For this review, take the finished solid that the model builds, in its own axes (mm). Coordinates: 2 decimals unless noted, no trailing zeros. Loops run counter-clockwise (first coordinate to the right, second up) from the corner with the lowest first, then second, coordinate; pieces in that order, holes last.
1. Take a section at A-A, the plane x = 3.4. State the section outline as (y, z) points, then the cut area to 3 significant figures.
2. Take a section at C-C, the plane y = 2.5. State the section outline as (x, z) points.
3. Clearance check with flat-ended pins moving along their axes: P1, Ø1, axis at y = -34.5, z = 51.5, coming from the -X side; P2, Ø1.5, axis at y = -28, z = -3.5, coming from the -X side; P3, Ø1.4, axis at x = 2, z = -3.5, coming from the +Y side; P4, Ø1.4, axis at x = 3, z = -2, coming from the -Y side. State where each tip first meets the part, or that it passes through.
4. Take a section at D-D, the plane y = 20.5. State the section outline as (x, z) points.
5. Take a section at B-B, the plane z = 77. State the section outline as (x, y) points, then the cut area to 3 significant figures.
6. To check wall thickness, follow probe 1 along Z at (x, y) = (2.8, 0); probe 2 along Z at (x, y) = (1.8, 8); probe 3 along Y at (x, z) = (3.8, 116). State the ranges of each line that lie inside material, in increasing order.
```python
from build123d import *

# Parameters (mm, degrees)
F0_W     = 5
F0_H     = 102
F1_DEPTH = 130
F2_SIZE2 = 100
F2_SIZE  = 35
F4_W     = 4.8
F4_H     = 19.5
F5_DEPTH = 5
F6_D     = 20.5
F7_D     = 20.5
F8_DEPTH = 25


# Not quite as in the source:
# - a feature names something its author has since deleted; it is built from what else it names


with BuildPart() as f1:
    # F0 (on Top) → F1 (new body)
    with BuildSketch(Plane.XY):
        with Locations((2.5, 0.1111116846)):
            Rectangle(F0_W, F0_H)
    extrude(amount=F1_DEPTH)

    # F2
    f2_edges = [f1.edges().sort_by_distance(p)[0] for p in [
        (2.5, -50.888888, 130),
        (2.5, 51.111112, 130),
    ]]
    f2_side = f1.faces().sort_by_distance((2.5, 0.111112, 130))[0]
    chamfer(f2_edges, length=F2_SIZE, length2=F2_SIZE2, reference=f2_side)

    # F4 (on face) → F5 (join)
    with BuildSketch(Plane(origin=(0, 0, 0), x_dir=(1, 0, 0), z_dir=(0, 0, -1))):
        with Locations((2.5, -25.1611116846)):
            Rectangle(F4_W, F4_H)
        with Locations((2.5, 24.9388883154)):
            Rectangle(F4_W, F4_H)
    extrude(amount=F5_DEPTH)

    # F6 (through all)
    with Locations(Plane(origin=(0, 0, 0), x_dir=(0, -1, 0), z_dir=(-1, 0, 0))):
        with Locations((-0.1111116846, 75)):
            Hole(F6_D / 2)

    # F7 (through all)
    with Locations(Plane(origin=(0, 0, 0), x_dir=(0, -1, 0), z_dir=(-1, 0, 0))):
        with Locations((0, 110)):
            Hole(F7_D / 2)

    # F3 (on face) → F8 (cut)
    with BuildSketch(Plane(origin=(0, 0, 0), x_dir=(0, -1, 0), z_dir=(-1, 0, 0))):
        Polygon((-28.4119545359, 79.7192917818), (-33.1312463177, 81.3710439055), (-36.434750565, 71.9324603418), (-31.7154587832, 70.2807082182), (-30.0637066595, 75), align=None)
        Polygon((28.1897311666, 79.7192917818), (29.8414832903, 75), (34.5607750721, 76.6517521236), (32.9090229484, 81.3710439055), align=None)
        Polygon((34.5607750721, 76.6517521236), (29.8414832903, 75), (31.4932354139, 70.2807082182), (36.2125271957, 71.9324603418), align=None)
    extrude(amount=-F8_DEPTH, mode=Mode.SUBTRACT)


solid = f1.part
```
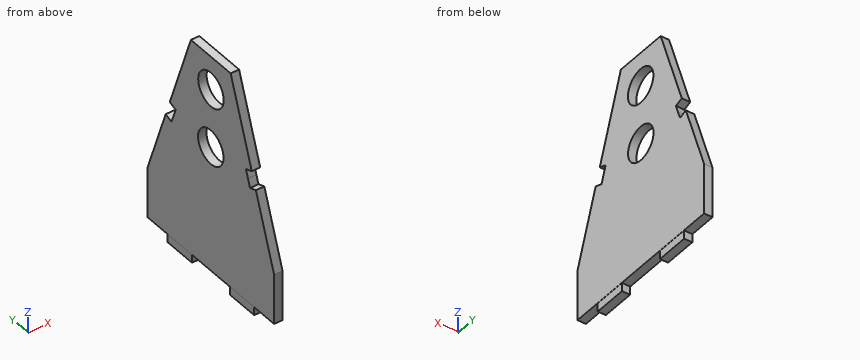
Results list:
1. outline: (-50.89, 0) - (-34.69, 0) - (-34.69, -5) - (-15.19, -5) - (-15.19, 0) - (15.41, 0) - (15.41, -5) - (34.91, -5) - (34.91, 0) - (51.11, 0) - (51.11, 30) - (36.43, 71.93) - (31.72, 70.28) - (28.41, 79.72) - (33.13, 81.37) - (16.11, 130) - (-15.89, 130) - (-32.91, 81.37) - (-28.19, 79.72) - (-31.49, 70.28) - (-36.21, 71.93) - (-50.89, 30) - close; hole circle Ø20.5 at (0, 110); hole circle Ø20.5 at (0.11, 75)
1. area: 9,190 mm2
2. outline: (0, 0) - (5, 0) - (5, 65.03) - (0, 65.03) - close; (0, 84.97) - (5, 84.97) - (5, 100.06) - (0, 100.06) - close; (0, 119.94) - (5, 119.94) - (5, 130) - (0, 130) - close
3. P1: stops at x = 0
3. P2: stops at x = 0.1
3. P3: stops at y = 34.91
3. P4: stops at y = -34.69
4. outline: (0, 0) - (0.1, 0) - (0.1, -5) - (4.9, -5) - (4.9, 0) - (5, 0) - (5, 117.46) - (0, 117.46) - close
5. outline: (0, -29.14) - (5, -29.14) - (5, -9.94) - (0, -9.94) - close; (0, 10.16) - (5, 10.16) - (5, 29.36) - (0, 29.36) - close
5. area: 192 mm2
6. probe 1: z = 0 to 64.75, 85.25 to 99.75, 120.25 to 130
6. probe 2: z = 0 to 68.46, 81.54 to 103.59, 116.41 to 130
6. probe 3: y = -20.79 to -8.31, 8.31 to 21.01
